Input: dimensioned drawing with shaded views. Units: mm. Origin: part minimum x, y, z. Give positions to 0.01 mm unless a question says otherwise; leave off trailing zeros. Order: outer loops, then holes, each group sorted by start corner. A loop starts at its lowest first (then second) coordinate and runs counter-clockwise, first axis right, second up. Notation, with made-up numbers: (67.25, -24.5) - (103.25, -24.5) arc R17 cw to (103.25, -13.5) - close; hole circle Ø11 at (54.5, 3.5). An arc over 180 degrees is marked (long way). Use a Markdown table: item, result.
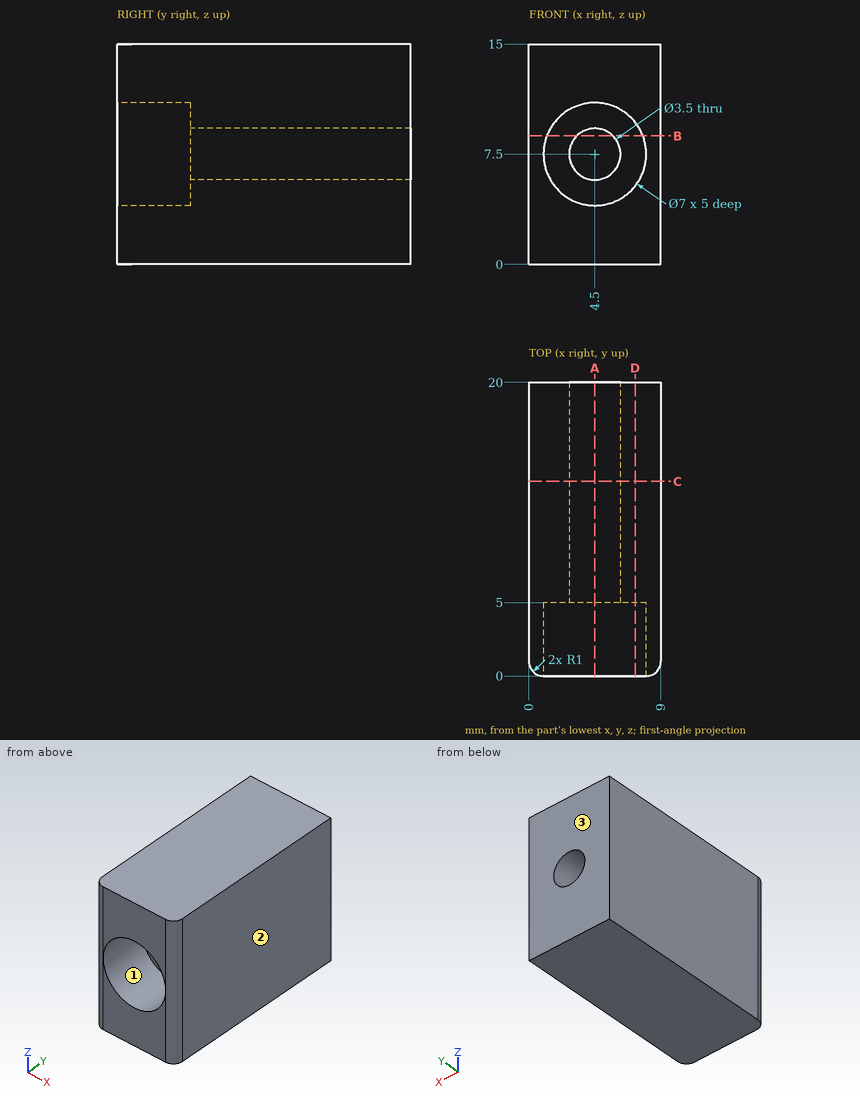
1. Material intervals for line 1 along Z through (x, y) = (4.5, 14.5); line 2 along Y through (x, z) = (6.75, 8); line 3 along Z through (x, y) = (4.5, 3.3), sorted ascending.
Response:
| item | result |
|---|---|
| line 1 | z = 0 to 5.75, 9.25 to 15 |
| line 2 | y = 5 to 20 |
| line 3 | z = 0 to 4, 11 to 15 |
2. Section query B-B (z = 8.75). Return loops of the section in (x, y).
Response:
| item | result |
|---|---|
| outline | (0, 1) arc R1 ccw to (1, 0) - (1.23, 0) - (1.23, 5) - (3.28, 5) - (3.28, 20) - (0, 20) - close; (5.72, 5) - (7.77, 5) - (7.77, 0) - (8, 0) arc R1 ccw to (9, 1) - (9, 20) - (5.72, 20) - close |
3. Section query A-A (x = 4.5). Return loops of the section in (y, z), then the cut area to 4 significant figures.
Response:
| item | result |
|---|---|
| outline | (0, 0) - (20, 0) - (20, 5.75) - (5, 5.75) - (5, 4) - (0, 4) - close; (0, 11) - (5, 11) - (5, 9.25) - (20, 9.25) - (20, 15) - (0, 15) - close |
| area | 212.5 mm^2 |
4. Section query D-D (x = 7.25). Return loops of the section in (y, z), then the cut area to 3 significant figures.
Response:
| item | result |
|---|---|
| outline | (0, 0) - (20, 0) - (20, 15) - (0, 15) - (0, 9.67) - (5, 9.67) - (5, 5.33) - (0, 5.33) - close |
| area | 278 mm^2 |
5. Pin query (flat end, axial travel): pin 1 (4 mm diameter, centred on x = 4.5, z = 7.5, fed in from -Y). Return the tip coordinate at first contact, or that it passes through.
Response:
| item | result |
|---|---|
| pin 1 | stops at y = 5 |
6. Mould query, pull axis X, two halves, no side actions, for the marked faces 1, 2 and 3. Classes: pulls with the +X half, pulls with the -X half, needs draft (parallel to the pull), parting line crosses it, or undercut.
Response:
| item | result |
|---|---|
| face 1 | undercut |
| face 2 | pulls with the +X half |
| face 3 | needs draft |
7. Section query C-C (y = 13.25). Return loops of the section in (x, z).
Response:
| item | result |
|---|---|
| outline | (0, 0) - (9, 0) - (9, 15) - (0, 15) - close; hole circle Ø3.5 at (4.5, 7.5) |
